Can you work these out from the model? Positions are in its coordinate system, mm. A direction names the side the tool comes from. Coordinates: 2 decimals unless noted, no trailing zeros. Loops run counter-clockwise (first coordinate to the right, second up) from the corner with the lowest first, then second, coordinate; pieces in that order, holes last.
```python
from build123d import *

# Parameters (mm, degrees)
SKETCH039_R            = 14.2875
SKETCH039_R_2          = 12.7
PAD036_DEPTH           = 29.21
SKETCH037_R            = 16.66875
SKETCH037_R_2          = 12.7
PAD041_DEPTH           = 12.7
SKETCH041_R            = 3.571875
PAD038_DEPTH           = 13
SKETCH040_R            = 34.528125
SKETCH040_R_2          = 14.2875
PAD037_DEPTH           = 12.7
CUT028_PLACEMENT_ANGLE = 60
CUT027_PLACEMENT_ANGLE = 60
CUT031_PLACEMENT_ANGLE = 60
CUT032_PLACEMENT_ANGLE = 60
CUT029_PLACEMENT_ANGLE = 60


with BuildPart() as body036:
    # Sketch039 → Pad036 (new body)
    with BuildSketch(Plane.XZ):
        Circle(SKETCH039_R)
        Circle(SKETCH039_R_2, mode=Mode.SUBTRACT)
    extrude(amount=PAD036_DEPTH)


with BuildPart() as body036_1:
    # Body036 placement: moved
    add(body036.part.moved(Location((0, -0.16, 0))))


with BuildPart() as body037:
    # Sketch037 → Pad041 (new body)
    with BuildSketch(Plane.XZ):
        Circle(SKETCH037_R)
        Circle(SKETCH037_R_2, mode=Mode.SUBTRACT)
    extrude(amount=PAD041_DEPTH)


with BuildPart() as body037_1:
    # Body037 placement: moved
    add(body037.part.moved(Location((0, -29.37, 0))))


with BuildPart() as body040:
    # Sketch041 → Pad038 (new body)
    with BuildSketch(Plane.XZ):
        with Locations((0, 29.36875)):
            Circle(SKETCH041_R)
    extrude(amount=PAD038_DEPTH)


with BuildPart() as fusion002:
    # Sketch040 → Pad037 (new body)
    with BuildSketch(Plane.XZ):
        Circle(SKETCH040_R)
        Circle(SKETCH040_R_2, mode=Mode.SUBTRACT)
    extrude(amount=PAD037_DEPTH)

    # Cut028: cut Body040
    add(body040.part, mode=Mode.SUBTRACT)


with BuildPart() as fusion002_1:
    # Cut028 placement: moved
    add(fusion002.part.rotate(Axis((0, 0, 0), (0, 1, 0)), CUT028_PLACEMENT_ANGLE))

    # Cut027: cut Body040
    add(body040.part, mode=Mode.SUBTRACT)


with BuildPart() as fusion002_2:
    # Cut027 placement: moved
    add(fusion002_1.part.rotate(Axis((0, 0, 0), (0, 1, 0)), CUT027_PLACEMENT_ANGLE))

    # Cut031: cut Body040
    add(body040.part, mode=Mode.SUBTRACT)


with BuildPart() as fusion002_3:
    # Cut031 placement: moved
    add(fusion002_2.part.rotate(Axis((0, 0, 0), (0, 1, 0)), CUT031_PLACEMENT_ANGLE))

    # Cut032: cut Body040
    add(body040.part, mode=Mode.SUBTRACT)


with BuildPart() as fusion002_4:
    # Cut032 placement: moved
    add(fusion002_3.part.rotate(Axis((0, 0, 0), (0, 1, 0)), CUT032_PLACEMENT_ANGLE))

    # Cut029: cut Body040
    add(body040.part, mode=Mode.SUBTRACT)


with BuildPart() as fusion002_5:
    # Cut029 placement: moved
    add(fusion002_4.part.rotate(Axis((0, 0, 0), (0, 1, 0)), CUT029_PLACEMENT_ANGLE))

    # Cut030: cut Body040
    add(body040.part, mode=Mode.SUBTRACT)

    # Fusion002: union Body036, Body037
    add(body036_1.part)
    add(body037_1.part)


solid = fusion002_5.part
```
(1) I want a section at D-D on z = 27. Write out the boundary of the cut face in (x, y), then the cut area to 3 significant figures.
Check values:
outline: (-21.52, -12.7) - (-2.67, -12.7) - (-2.67, 0) - (-21.52, 0) - close; (2.67, -12.7) - (21.52, -12.7) - (21.52, 0) - (2.67, 0) - close
area: 479 mm2
(2) I'm going to push flat-ended pins straight in: pin 1 (1 mm diameter, centred on x = 9, y = -19.5, fed in from -Z); pin 2 (8 mm diameter, centred on x = -25.43, z = 14.68, fed in from -Y); pin 3 (5 mm diameter, centred on x = 3.5, y = -31.5, fed in from -Z). Where does each tip first touch, or does it pass through?
Check values:
pin 1: stops at z = -11.48
pin 2: stops at y = -12.7
pin 3: stops at z = -16.64
(3) Which directions (+Z, -Z, +X, -X, +Y, -Y) give clear straight access to the entire face, cutting with the end or side of a thin tool? Please do faces 1 (the flat face through (-13, -0.16, -1)), 2 (the flat face through (7, -12.7, 13)), 3 (the cylindrical face through (15.9, -35.6, 5)).
Check values:
face 1: +Y
face 2: none
face 3: -Y
(4) If we mould it in two halves opening along Z, with no side actions, what happens to faces 4 (the cylindrical face through (13.63, -20.92, 4.29)), 5 (the cylindrical face through (22.135, -6.261, 16.052)), 6 (the cylindrical face through (-2.75, -20.82, -12.4)), 7 (the flat face through (7, 0, 13))? For each: released by +Z, released by -Z, zero draft, split by the parting line, or undercut.
Check values:
face 4: split by the parting line
face 5: undercut
face 6: undercut
face 7: zero draft
(5) I want a section at A-A on z = 0. Write out the boundary of the cut face in (x, y).
Check values:
outline: (-34.53, -12.7) - (-14.29, -12.7) - (-14.29, -29.37) - (-16.67, -29.37) - (-16.67, -42.07) - (-12.7, -42.07) - (-12.7, -0.16) - (-14.29, -0.16) - (-14.29, 0) - (-34.53, 0) - close; (12.7, -42.07) - (16.67, -42.07) - (16.67, -29.37) - (14.29, -29.37) - (14.29, -12.7) - (34.53, -12.7) - (34.53, 0) - (14.29, 0) - (14.29, -0.16) - (12.7, -0.16) - close
(6) I want a section at C-C on y = -17.5. Write out the boundary of the cut face in (x, z) (1 decimal).
Check values:
outline: circle Ø28.6 at (0, 0); hole circle Ø25.4 at (0, 0)
(7) If I drill on probe 1 along X at (y, z) = (-7, -0.5); probe 2 along Z at (x, y) = (-22.5, -7.5); probe 3 along Y at (x, z) = (-16, -9.5), over which ranges is the centre line in solid material (lowest first)?
Check values:
probe 1: x = -34.52 to -12.69, 12.69 to 34.52
probe 2: z = -26.19 to -16.72, -12.65 to 12.65, 16.72 to 26.19
probe 3: y = -12.7 to 0
(8) I want a section at B-B on x = 0. Write out the boundary of the cut face in (y, z), then the cut area to 3 significant figures.
Check values:
outline: (-42.07, -16.67) - (-29.37, -16.67) - (-29.37, -14.29) - (-12.7, -14.29) - (-12.7, -25.8) - (0, -25.8) - (0, -14.29) - (-0.16, -14.29) - (-0.16, -12.7) - (-42.07, -12.7) - close; (-42.07, 12.7) - (-0.16, 12.7) - (-0.16, 14.29) - (0, 14.29) - (0, 25.8) - (-12.7, 25.8) - (-12.7, 14.29) - (-29.37, 14.29) - (-29.37, 16.67) - (-42.07, 16.67) - close; (-12.7, -34.53) - (0, -34.53) - (0, -32.94) - (-12.7, -32.94) - close; (-12.7, 32.94) - (0, 32.94) - (0, 34.53) - (-12.7, 34.53) - close
area: 526 mm2
